Source: CAD feature listing. Evaluate the final solid. Frame: model axes, mm. Face numbers are marked on the shaded views. Give positions to 0.01 mm unless a question says otherwise; leave off trailing zeros. Order: outer loops, then holes, each group sorted by start corner. A loop starts at its lowest first (then second) coordinate and runs counter-clockwise, first axis right, second up. Notation, with made-up numbers: (3, -16) -> (9, -16) arc R34 cw to (9, 20) -> close; hole circle Ø5 at (-15, 37). An arc over 180 degrees is marked (long way). Use one line per item in the form item = value. Start each with the question number.
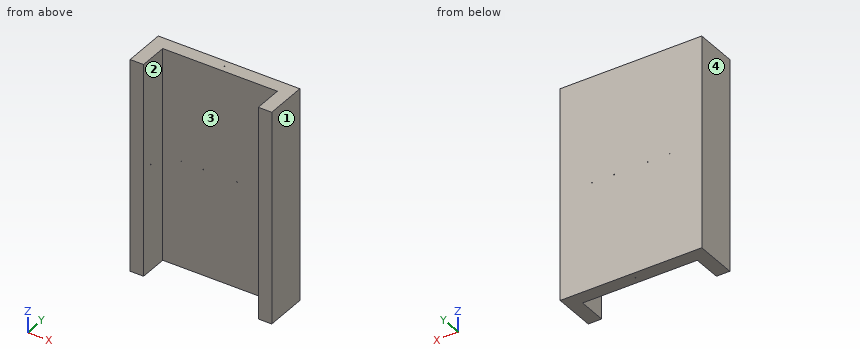
from build123d import *

# Parameters (mm, degrees)
F0_W      = 200
F0_H      = 300
F0_R      = 0.5
F1_DEPTH  = 19
F2_W      = 19
F2_H      = 300
F3_DEPTH  = 40.5
F4_R      = 0.5
F5_DEPTH  = 1
F6_R      = 0.5
F7_DEPTH  = 1
F8_R      = 0.5
F9_DEPTH  = 1
F10_R     = 0.5
F11_DEPTH = 1


with BuildPart() as f1:
    # F0 (on Front) → F1 (new body)
    with BuildSketch(Plane.XZ):
        with Locations((100, 150)):
            Rectangle(F0_W, F0_H)
        with Locations((45, 150)):
            Circle(F0_R, mode=Mode.SUBTRACT)
        with Locations((76.153976, 150)):
            Circle(F0_R, mode=Mode.SUBTRACT)
        with Locations((123.846024, 150)):
            Circle(F0_R, mode=Mode.SUBTRACT)
        with Locations((155, 150)):
            Circle(F0_R, mode=Mode.SUBTRACT)
    extrude(amount=F1_DEPTH)

    # F2 (on face) → F3 (join)
    with BuildSketch(Plane.XZ.offset(19)):
        with Locations((9.5, 150)):
            Rectangle(F2_W, F2_H)
        with Locations((190.5, 150)):
            Rectangle(F2_W, F2_H)
    extrude(amount=F3_DEPTH)

    # F4 (on face) → F5 (cut)
    with BuildSketch(Plane.YZ.offset(19)):
        with Locations((-44.5, 150)):
            Circle(F4_R)
    extrude(amount=-F5_DEPTH, mode=Mode.SUBTRACT)

    # F6 (on face) → F7 (cut)
    with BuildSketch(Plane(origin=(181, 0, 0), x_dir=(0, -1, 0), z_dir=(-1, 0, 0))):
        with Locations((44.5, 150)):
            Circle(F6_R)
    extrude(amount=-F7_DEPTH, mode=Mode.SUBTRACT)

    # F8 (on face) → F9 (cut)
    with BuildSketch(Plane(origin=(0, 0, 0), x_dir=(1, 0, 0), z_dir=(0, 0, -1))):
        with Locations((100, 9.5)):
            Circle(F8_R)
    extrude(amount=-F9_DEPTH, mode=Mode.SUBTRACT)

    # F10 (on face) → F11 (cut)
    with BuildSketch(Plane.XY.offset(300)):
        with Locations((100, -9.5)):
            Circle(F10_R)
    extrude(amount=-F11_DEPTH, mode=Mode.SUBTRACT)


solid = f1.part
1) Pin query (flat end, axial travel): pin 1 (4 mm diameter, centred on x = 29.5, z = 94, fed in from -Y); pin 2 (0.5 mm diameter, centred on x = 100, y = -9.5, fed in from -Z). Return the tip coordinate at first contact, or that it passes through.
2) Material intervals for probe 1 along X at (y, z) = (-11, 150); probe 2 along Y at (x, z) = (100, 299.65); probe 3 along Y at (x, z) = (181.3, 150), sorted ascending.
3) Cut plane B-B, the plane y = -22.5. Return the cut outline in (x, z), plus the area to 3 significant figures.
4) Draft query along X for the marked faces 1, 2, 3 and 4. Return one class per face: +X half, -X half, draft (parallel to the pull), parting line (faces both ways), or undercut.
5) Cut plane C-C, the plane x = 65. Return the cut outline in (y, z), plus the area to 3 significant figures.
6) Cut plane A-A, the plane z = 238.5. Return the cut outline in (x, y), plus the area to 3 significant figures.
Output values:
q1.pin_1 = -19
q1.pin_2 = 1
q2.probe_1 = 0 to 44.5, 45.5 to 75.65, 76.65 to 123.35, 124.35 to 154.5, 155.5 to 200
q2.probe_2 = -19 to -10, -9 to 0
q2.probe_3 = -59.5 to -45, -44 to 0
q3.outline = (0, 0) -> (19, 0) -> (19, 300) -> (0, 300) -> close; (181, 0) -> (200, 0) -> (200, 300) -> (181, 300) -> close
q3.area = 11,400 mm^2
q4.face_1 = +X half
q4.face_2 = undercut
q4.face_3 = undercut
q4.face_4 = -X half
q5.outline = (-19, 0) -> (0, 0) -> (0, 300) -> (-19, 300) -> close
q5.area = 5,700 mm^2
q6.outline = (0, -59.5) -> (19, -59.5) -> (19, -19) -> (181, -19) -> (181, -59.5) -> (200, -59.5) -> (200, 0) -> (0, 0) -> close
q6.area = 5,340 mm^2
